The listing builds one solid part. Answer for the finished solid, in the listing's coordinates (mm). A direction names the side the tool comes from. Round coordinates to 2 decimals unless told otherwise and drop trailing zeros. Order: outer loops, then holes, each group sorted by start corner. A loop starts at its lowest first (then second) coordinate and runs counter-clockwise, first axis right, second up. Notation, with made-up numbers: (-21.75, 4.25) - (5.25, 4.25) arc R23 cw to (5.25, 42.25) - close; hole circle Ø9 at (30.5, 68.25). An arc over 180 degrees is marked (long way). One line per item, written item: value. Start each with the question number.
1. Section B-B, the plane z = 0 is taken. Give the vertices of the cut face in (x, y).
2. Section A-A, the plane x = 29.75 is taken. Give the vertices of the cut face in (y, z).
3. Section D-D, the plane y = 99.5 is taken. Give the vertices of the cut face in (x, z).
4. Section C-C, the plane y = 93 is taken. Give the vertices of the cut face in (x, z).
5. For a pull along Z with two mould halves and no side action, classify faces 6 (the flat face through (31, 109.5, 3)), 7 (the cylindrical face through (29.486, 97.175, 5.994)), 8 (the cylindrical face through (29.651, 92.825, 2.248)) as released by +Z, released by -Z, zero draft, split by the parting line, or undercut.
6. Flat-ended cylindrical pins translate along their axes: P1, Ø5, axis at y = 86, z = 4, coming from the +X side; P2, Ø3, axis at y = 93.5, z = 4, coming from the -X side; P3, Ø5, axis at x = 32.5, y = 91.5, coming from the +Z side. Find the tip coordinate at first contact, or state that the pin passes through.
7. Straight lines are drawn through the part: line 1 (Z direction, x = 29.75, y = 88.75); line 2 (Y direction, x = 29.25, z = 1.75); line 3 (X direction, y = 99.5, z = -3.3). For each, find the intervals that lie inside material, in ascending order.
8. A tool of negligible diameter and unlimited length cuts with its end or side. For faces 1 (the flat face through (32, 80.5, 1)), 2 (the flat face through (30, 105.5, 0)), 3 (the cylindrical face through (32.68, 111.02, 0.65)), 4 (the flat face through (30, 112.5, 0)), 5 (the cylindrical face through (31.3, 98.8, -3.2)), from which of +Z, -Z, +X, -X, +Y, -Y can it reach the whole face along a straight path? Write none if from no direction.
from build123d import *

# Parameters (mm, degrees)
REBAIXO_PARA_SBHCS_M36_D           = 3.4
REBAIXO_PARA_SBHCS_M36_DEPTH       = 5
REBAIXO_PARA_SBHCS_M36_CBORE_D     = 6.7
REBAIXO_PARA_SBHCS_M36_CBORE_DEPTH = 1.65
REBAIXO_PARA_SBHCS_M36_TIP         = 1.021463052


with BuildPart() as part:
    # Esboço1 → Revolução1 (revolve)
    with BuildSketch(Plane.XY, mode=Mode.PRIVATE) as revolu_o1_sk:
        Polygon((29.75, 112.5), (29.75, 105.5), (32, 105.5), (32, 80.5), (34.5, 80.5), (35.75, 84.5), (35.75, 109.5), (32.75, 109.5), (32.75, 112.5), align=None)
    revolve(revolu_o1_sk.sketch.rotate(Axis((29.75, 33.489540419, 0), (0, 1, 0)), 90), axis=Axis((29.75, 33.489540419, 0), (0, 1, 0)))

    # Rebaixo para SBHCS M36
    with Locations(Plane(origin=(0, 0, -6), x_dir=(-1, 0, 0), z_dir=(0, 0, -1))):
        with Locations((-29.75, 99.5)):
            CounterBoreHole(REBAIXO_PARA_SBHCS_M36_D / 2, REBAIXO_PARA_SBHCS_M36_CBORE_D / 2, REBAIXO_PARA_SBHCS_M36_CBORE_DEPTH, depth=REBAIXO_PARA_SBHCS_M36_DEPTH)
            with Locations((0, 0, -(REBAIXO_PARA_SBHCS_M36_DEPTH + REBAIXO_PARA_SBHCS_M36_TIP / 2))):  # 118° drill point
                Cone(0, REBAIXO_PARA_SBHCS_M36_D / 2, REBAIXO_PARA_SBHCS_M36_TIP, mode=Mode.SUBTRACT)


solid = part.part
Answer list:
1. outline: (23.75, 84.5) - (25, 80.5) - (27.5, 80.5) - (27.5, 105.5) - (32, 105.5) - (32, 80.5) - (34.5, 80.5) - (35.75, 84.5) - (35.75, 109.5) - (32.75, 109.5) - (32.75, 112.5) - (26.75, 112.5) - (26.75, 109.5) - (23.75, 109.5) - close
2. outline: (80.5, -4.75) - (84.5, -6) - (96.15, -6) - (96.15, -4.35) - (97.8, -4.35) - (97.8, -2.25) - (80.5, -2.25) - close; (80.5, 2.25) - (105.5, 2.25) - (105.5, -2.25) - (101.2, -2.25) - (101.2, -4.35) - (102.85, -4.35) - (102.85, -6) - (109.5, -6) - (109.5, -3) - (112.5, -3) - (112.5, 3) - (109.5, 3) - (109.5, 6) - (84.5, 6) - (80.5, 4.75) - close
3. outline: (26.4, -4.98) - (26.4, -4.35) - (28.05, -4.35) - (28.05, -1.47) arc R2.25 cw (long way) to (31.45, -1.47) - (31.45, -4.35) - (33.1, -4.35) - (33.1, -4.98) arc R6 ccw (long way) to start
4. outline: circle Ø12 at (29.75, 0); hole circle Ø4.5 at (29.75, 0)
5. face 6: zero draft
5. face 7: split by the parting line
5. face 8: undercut
6. P1: stops at x = 35.56
6. P2: stops at x = 24.3
6. P3: stops at z = 5.99
7. line 1: z = -6 to -2.25, 2.25 to 6
7. line 2: y = 105.5 to 112.5
7. line 3: x = 24.74 to 28.05, 31.45 to 34.76
8. face 1: +Z, -Z, +X, -X, -Y
8. face 2: -Y
8. face 3: +Y
8. face 4: +Z, -Z, +X, -X, +Y
8. face 5: -Z
